Solid Edge part; units mm, degrees
sketch "Sketch1" plane through (0, 0, 0) normal (0, 0, 1) x (1, 0, 0)
  line L0 (0, 0) -> (-204.46, 0)
  line L1 (-204.46, 0) -> (-204.46, -94)
  line L2 (-204.46, -94) -> (0, -94)
  line L3 (0, -94) -> (0, 0)
extrude "Protrusion1" add sketch "Sketch1" against normal blind 20.2
sketch "Sketch2" plane through (-102.23, -47, 0) normal (0, 0, 1) x (1, 0, 0)
  circle A0 centre (42, 7) radius 6.5
  circle A1 centre (-42, 7) radius 6.5
extrude "ExtrudedCutout_1" cut sketch "Sketch2" against normal blind 21
sketch "Sketch3" plane through (-102.23, -47, 0) normal (0, 0, 1) x (1, 0, 0)
  circle A0 centre (-125, -9.55) radius 55
extrude "ExtrudedCutout_2" cut sketch "Sketch3" against normal blind 22
sketch "Sketch4" plane through (-102.23, -47, 0) normal (0, 0, 1) x (1, 0, 0)
  circle A0 centre (125, -9.55) radius 55
extrude "ExtrudedCutout_3" cut sketch "Sketch4" against normal blind 22
fillet "Round_1" radius 3 2 edges at (0, 0, -10.1) (-204.46, 0, -10.1)
The listing builds one solid part. Answer for the finished solid, in the listing's coordinates (mm). Coordinates: 2 decimals unless noted, no trailing zeros. Order: outer loops, then holes, each group sorted by start corner. A loop starts at its lowest first (then second) coordinate and runs counter-clockwise, first axis right, second up. Notation, with made-up numbers: M 40,44 L 54,44 A31 cw 54,68 Z; hole C -32.5,-33.75 d6. An arc over 180 degrees is marked long. Answer as a JSON object with one key per item and string values. Group by question number.
1. Section D-D on y = -60 is taken. Write down the section's boundary in (x, z).
2. Determine the mould class of faces 1 (the flat face through (-101, 0, -10)), 2 (the cylindrical face through (-31.013, -45.046, -9.959)), 3 (the flat face through (-104, -46, -20.2)), 4 (the cylindrical face through (-138.03, -38.05, -9.96)) for opening direction Y: released by +Y, released by -Y, zero draft, split by the parting line, or undercut.
3. Section A-A on x = -60.23 is taken. Write down the section's boundary in (y, z), then the cut area to 3 significant figures.
4. Flat-ended cylindrical pins translate along their axes: P1, Ø15, axis at x = -144.23, y = -40, coming from the -Z side; P2, Ø10, axis at y = -29, z = -5, coming from the +X side; P3, Ø10, axis at y = -30, z = -8.5, coming from the -X side; P4, Ø8, axis at x = -60.23, y = -40, coming from the +Z side. Find the tip coordinate at first contact, or state that the pin passes through.
5. Section B-B on z = -3.5 is taken. Write down the section's boundary in (x, y).
6. Straight lines are drawn through the part: line 1 (Y direction, x = -144.23, z = -8); line 2 (X direction, y = -39, z = -8); line 3 (X direction, y = -44, z = -15.5). For each, find the intervals that lie inside material, in ascending order.
7. Section C-C on y = -40 is taken. Write down the section's boundary in (x, z).
Values follow:
{
 "1": {"outline": "M -172.34,-20.2 L -32.12,-20.2 L -32.12,0 L -172.34,0 Z"},
 "2": {"face 1": "released by +Y", "face 2": "undercut", "face 3": "zero draft", "face 4": "undercut"},
 "3": {"outline": "M -94,-20.2 L -46.5,-20.2 L -46.5,0 L -94,0 Z; M -33.5,-20.2 L 0,-20.2 L 0,0 L -33.5,0 Z", "area": "1,640 mm2"},
 "4": {"P1": "z = -20.2", "P2": "x = -21.56", "P3": "x = -182.18", "P4": "through"},
 "5": {"outline": "M -204.46,-6.48 A55 cw -186.95,-94 L -17.51,-94 A55 cw 0,-6.48 L 0,-3 A3 ccw -3,0 L -201.46,0 A3 ccw -204.46,-3 Z; hole C -144.23,-40 d13; hole C -60.23,-40 d13"},
 "6": {"line 1": "-94 to -46.5, -33.5 to 0", "line 2": "-175.11 to -150.65, -137.81 to -66.65, -53.81 to -29.35", "line 3": "-173.68 to -149.35, -139.11 to -65.35, -55.11 to -30.78"},
 "7": {"outline": "M -174.78,-20.2 L -150.73,-20.2 L -150.73,0 L -174.78,0 Z; M -137.73,-20.2 L -66.73,-20.2 L -66.73,0 L -137.73,0 Z; M -53.73,-20.2 L -29.68,-20.2 L -29.68,0 L -53.73,0 Z"}
}
